Answer from the drawing. Dimensions are ordinates in mm from the lowest x, y and z of the part. Give positions to 0.01 mm unless a question says otherwise; leave off trailing zeros. Loops run counter-clockwise (first coordinate to the right, second up) from the corner with the lowest first, then second, coordinate; pieces in that order, holes last.
(1) Find section B-B, the plane x = 1.5. Write down the section's boundary in (y, z), then the cut area to 3 significant figures.
(2) Each of these flat-tipped pins is pushed along its axis until it touches: P1, Ø1.5, axis at x = 1.5, y = 4.5, coming from the -Z side; P2, Ø4, axis at y = 1, z = 7, coming from the -X side; P3, Ø5, axis at x = 8, z = 35, coming from the +Y side; P4, Ø3, axis at x = 4.9, y = 4.9, coming from the -Z side. Where does it stop, or does it pass through?
(3) Find section A-A, the plane z = 4. Write down the section's boundary in (x, y).
(4) Find section C-C, the plane z = 13. Write down the section's boundary in (x, y).
(5) Find section D-D, the plane y = 8.5. Write down the section's boundary in (x, z) (1 decimal).
(6) Straight lines are drawn through the part: probe 1 along X at (y, z) = (5, 39); probe 2 along Y at (x, z) = (3.5, 11) (1 decimal). For each, find the intervals that lie inside material, in ascending order.
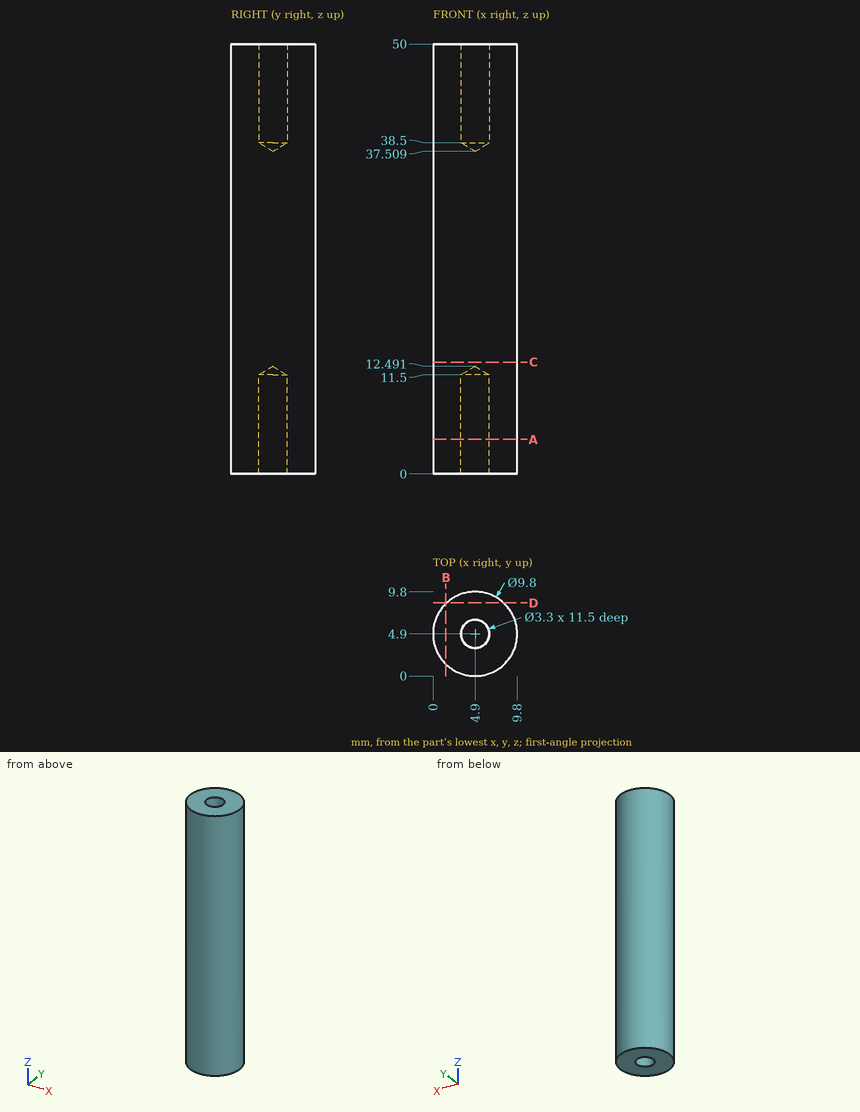
Entries:
1. outline: (1.37, 0) - (8.43, 0) - (8.43, 50) - (1.37, 50) - close
1. area: 353 mm2
2. P1: stops at z = 0
2. P2: stops at x = 0.38
2. P3: stops at y = 9.76
2. P4: stops at z = 11.59
3. outline: circle Ø9.8 at (4.9, 4.9); hole circle Ø3.3 at (4.9, 4.9)
4. outline: circle Ø9.8 at (4.9, 4.9)
5. outline: (1.6, 0) - (8.2, 0) - (8.2, 50) - (1.6, 50) - close
6. probe 1: x = 0 to 3.25, 6.55 to 9.8
6. probe 2: y = 0.2 to 4, 5.8 to 9.6
